Design review of the part built by this model. Coordinates are the model's own, in mm. A direction names the side the tool comes from. Coordinates: 2 decimals unless noted, no trailing zeros. Write each loop counter-clockwise with the first axis right and the second up, starting at its lowest first coordinate (ties: lowest second). Pieces come first, ordered by that corner, then holes.
Q1. Add section C-C, the plane z = -7.5. Give the boundary of the cut face in (x, y).
Q2. Add section A-A, the plane y = 31. Give the boundary of the cut face in (x, z), plus the area to 3 significant figures.
Q3. To check wall thickness, follow probe 1 along Y at (x, z) = (13.9, -7.5); probe 2 along Y at (x, z) = (7.5, -14); probe 3 along Z at (x, y) = (10.5, 30). State the ranges of each line that lie inside material, in increasing order.
Q4. Add section B-B, the plane x = 7.5. Give the boundary of the cut face in (y, z).
Q5. The part is to be moulded in two halves that separate along Z. For faces 1 (the face through (0.74, 34.536, -7.825)), 2 (the face through (9, 11, -1)), 3 (the face through (1, 6, -9)), 4 (the face through (7, 21, -15)), say which applies: +Z half, -Z half, draft (parallel to the pull), parting line (faces both ways), or undercut.
Q6. Add section D-D, the plane x = 9.5. Give the boundary of the cut face in (y, z).
Q7. Machinability: for faces 5 (the face through (13.5, 21, -7)), 6 (the face through (14.24, 34.536, -7.825)), which of the approach directions +Z, -Z, +X, -X, +Y, -Y give a long, thin tool a straight path to every point of the face, cutting with its end or side? Answer none if there is none.
from build123d import *

# Parameters (mm, degrees)
SKETCH1_W           = 15
SKETCH1_H           = 15
SKETCH1_W_2         = 12
SKETCH1_H_2         = 12
EXTRUDE_THIN1_DEPTH = 42
SKETCH2_R           = 1.5
CUT_EXTRUDE1_DEPTH  = 16
SKETCH3_R           = 1.5
CUT_EXTRUDE2_DEPTH  = 16


with BuildPart() as part:
    # Sketch1 → Extrude-Thin1 (new body)
    with BuildSketch(Plane(origin=(0, 0, 0), x_dir=(1, 0, 0), z_dir=(0, 1, 0))):
        with Locations((7.5, 7.5)):
            Rectangle(SKETCH1_W, SKETCH1_H)
        with Locations((7.5, 7.5)):
            Rectangle(SKETCH1_W_2, SKETCH1_H_2, mode=Mode.SUBTRACT)
    extrude(amount=EXTRUDE_THIN1_DEPTH)

    # Sketch2 → Cut-Extrude1 (cut, through all)
    with BuildSketch(Plane.ZY):
        with Locations((-7.5, 36)):
            Circle(SKETCH2_R)
        with Locations((-7.5, 6)):
            Circle(SKETCH2_R)
    extrude(amount=-CUT_EXTRUDE1_DEPTH, mode=Mode.SUBTRACT)

    # Sketch3 → Cut-Extrude2 (cut, through all)
    with BuildSketch(Plane(origin=(0, 0, -15), x_dir=(-1, 0, 0), z_dir=(0, 0, -1))):
        with Locations((-7.5, 31)):
            Circle(SKETCH3_R)
        with Locations((-7.5, 11)):
            Circle(SKETCH3_R)
    extrude(amount=-CUT_EXTRUDE2_DEPTH, mode=Mode.SUBTRACT)


solid = part.part
Here are the results:
1. outline: (0, 0) - (1.5, 0) - (1.5, 4.5) - (0, 4.5) - close; (0, 7.5) - (1.5, 7.5) - (1.5, 34.5) - (0, 34.5) - close; (0, 37.5) - (1.5, 37.5) - (1.5, 42) - (0, 42) - close; (13.5, 0) - (15, 0) - (15, 4.5) - (13.5, 4.5) - close; (13.5, 7.5) - (15, 7.5) - (15, 34.5) - (13.5, 34.5) - close; (13.5, 37.5) - (15, 37.5) - (15, 42) - (13.5, 42) - close
2. outline: (0, -15) - (6, -15) - (6, -13.5) - (1.5, -13.5) - (1.5, -1.5) - (6, -1.5) - (6, 0) - (0, 0) - close; (9, -15) - (15, -15) - (15, 0) - (9, 0) - (9, -1.5) - (13.5, -1.5) - (13.5, -13.5) - (9, -13.5) - close
2. area: 72.0 mm2
3. probe 1: y = 0 to 4.5, 7.5 to 34.5, 37.5 to 42
3. probe 2: y = 0 to 9.5, 12.5 to 29.5, 32.5 to 42
3. probe 3: z = -15 to -13.5, -1.5 to 0
4. outline: (0, -15) - (9.5, -15) - (9.5, -13.5) - (0, -13.5) - close; (0, -1.5) - (9.5, -1.5) - (9.5, 0) - (0, 0) - close; (12.5, -15) - (29.5, -15) - (29.5, -13.5) - (12.5, -13.5) - close; (12.5, -1.5) - (29.5, -1.5) - (29.5, 0) - (12.5, 0) - close; (32.5, -15) - (42, -15) - (42, -13.5) - (32.5, -13.5) - close; (32.5, -1.5) - (42, -1.5) - (42, 0) - (32.5, 0) - close
5. face 1: undercut
5. face 2: draft
5. face 3: undercut
5. face 4: -Z half
6. outline: (0, -15) - (42, -15) - (42, -13.5) - (0, -13.5) - close; (0, -1.5) - (42, -1.5) - (42, 0) - (0, 0) - close
7. face 5: +Y, -Y
7. face 6: +X, -X
